```python
from build123d import *

# Parameters (mm, degrees)
SKETCH1_R            = 5
SKETCH1_R_2          = 4
BOSS_EXTRUDE1_DEPTH  = 289.5
M3_CLEARANCE_HOLE1_D = 3.2


with BuildPart() as part:
    # Sketch1 → Boss-Extrude1 (new, symmetric)
    with BuildSketch(Plane(origin=(0, 0, 0), x_dir=(1, 0, 0), z_dir=(0, 1, 0))):
        Circle(SKETCH1_R)
        Circle(SKETCH1_R_2, mode=Mode.SUBTRACT)
    extrude(amount=BOSS_EXTRUDE1_DEPTH, both=True)

    # M3 Clearance Hole1 (through all)
    with Locations(Plane.ZY.offset(5)):
        with Locations((0, -284.5)):
            m3_clearance_hole1 = Hole(M3_CLEARANCE_HOLE1_D / 2)

    # Mirror1: M3 Clearance Hole1 across plane
    add(m3_clearance_hole1.mirror(Plane.ZX), mode=Mode.SUBTRACT)


solid = part.part
```
Could you check a few things on this model? Use its own coordinates, in mm. Give positions to 0.01 mm unless a question says otherwise; leave off trailing zeros. Order: outer loops, then holes, each group sorted by start corner. A loop starts at its lowest first (then second) coordinate and runs counter-clockwise, first axis right, second up.
Q1. Suppose I cut it at B-B, the plane z = 0. Write out the boundary of the cut face in (x, y), and give its area (3 significant figures).
Q2. Suppose I cut it at C-C, the plane y = 182.5. Write out the boundary of the cut face in (x, z), and give its area (3 significant figures).
Q3. If I drill on line 1 along Y through (x, z) = (-4.45, 0); line 2 along X through (y, z) = (-15.5, -0.5); line 3 along X through (y, z) = (254, 0.75), over which ranges is the centre line in solid material (lowest first)?
Q4. Suppose I cut it at A-A, the plane x = 0. Write out the boundary of the cut face in (y, z), and give its area (3 significant figures).
Q5. I'm going to push flat-ended pins straight in: P1, Ø1.5, axis at x = -3.5, y = -204.5, coming from the -Z side; P2, Ø1, axis at x = -1.5, y = -156, coming from the +Z side. Where does each tip first touch, or does it pass through?
Solution:
1. outline: (-5, -289.5) - (-4, -289.5) - (-4, -286.1) - (-5, -286.1) - close; (-5, -282.9) - (-4, -282.9) - (-4, 282.9) - (-5, 282.9) - close; (-5, 286.1) - (-4, 286.1) - (-4, 289.5) - (-5, 289.5) - close; (4, -289.5) - (5, -289.5) - (5, -286.1) - (4, -286.1) - close; (4, -282.9) - (5, -282.9) - (5, 282.9) - (4, 282.9) - close; (4, 286.1) - (5, 286.1) - (5, 289.5) - (4, 289.5) - close
1. area: 1,150 mm2
2. outline: circle Ø10 at (0, 0); hole circle Ø8 at (0, 0)
2. area: 28.3 mm2
3. line 1: y = -289.5 to -286.1, -282.9 to 282.9, 286.1 to 289.5
3. line 2: x = -4.97 to -3.97, 3.97 to 4.97
3. line 3: x = -4.94 to -3.93, 3.93 to 4.94
4. outline: (-289.5, -5) - (289.5, -5) - (289.5, -4) - (-289.5, -4) - close; (-289.5, 4) - (289.5, 4) - (289.5, 5) - (-289.5, 5) - close
4. area: 1,160 mm2
5. P1: stops at z = -4.18
5. P2: stops at z = 4.9
